Input: part model. Units: mm. Frame: model coordinates. A direction names the side the tool comes from. Coordinates: 2 decimals unless noted, no trailing zeros. Order: outer loops, then holes, each group sorted by start corner. A loop starts at its lowest first (then second) coordinate and runs counter-clockwise, first axis right, second up. Notation, with made-up numbers: (22.25, -25) -> (68.25, -25) arc R37 ccw to (68.25, 14) -> close; hole circle Ø11 at (-17.5, -34). An arc over 180 degrees is marked (long way). One line per question, with ' | ' between items.
```python
from build123d import *

# Parameters (mm, degrees)
F0_W      = 22.5
F0_H      = 11.8
F1_DEPTH  = 22.7
F2_W      = 4.7
F2_H      = 2.5
F3_DEPTH  = 11.8
F5_DEPTH  = 2.5
F7_DEPTH  = 2.5
F9_DEPTH  = 4
F10_R     = 2.3
F10_R_2   = 0.85
F11_DEPTH = 3.2
F13_DEPTH = 2


with BuildPart() as f1:
    # F0 (on Top) → F1 (new body)
    with BuildSketch(Plane.XY):
        with Locations((-42.3355284333, 9.1565789297)):
            Rectangle(F0_W, F0_H)
    extrude(amount=F1_DEPTH)

    # F2 (on face) → F3 (join)
    with BuildSketch(Plane.XZ.offset(-3.2565789297)):
        with Locations((-55.9355284333, 17.15)):
            Rectangle(F2_W, F2_H)
        with Locations((-28.7355284333, 17.15)):
            Rectangle(F2_W, F2_H)
    extrude(amount=-F3_DEPTH)

    # F4 (on face) → F5 (cut)
    with BuildSketch(Plane.XY.offset(18.4)):
        with BuildLine():
            Line((-58.2855284333, 8.5065789297), (-56.745462641, 8.5065789297))
            ThreePointArc((-56.745462641, 8.5065789297), (-54.9855284333, 9.1565789297), (-56.745462641, 9.8065789297))
            Line((-56.745462641, 9.8065789297), (-58.2855284333, 9.8065789297))
            Line((-58.2855284333, 9.8065789297), (-58.2855284333, 9.1565789297))
            Line((-58.2855284333, 9.1565789297), (-58.2855284333, 8.5065789297))
        make_face()
    extrude(amount=-F5_DEPTH, mode=Mode.SUBTRACT)

    # F6 (on face) → F7 (cut)
    with BuildSketch(Plane.XY.offset(18.4)):
        with BuildLine():
            Line((-26.3855284333, 9.8065789297), (-27.9255942256, 9.8065789297))
            ThreePointArc((-27.9255942256, 9.8065789297), (-29.6855284333, 9.1565789297), (-27.9255942256, 8.5065789297))
            Line((-27.9255942256, 8.5065789297), (-26.3855284333, 8.5065789297))
            Line((-26.3855284333, 8.5065789297), (-26.3855284333, 9.1565789297))
            Line((-26.3855284333, 9.1565789297), (-26.3855284333, 9.8065789297))
        make_face()
    extrude(amount=-F7_DEPTH, mode=Mode.SUBTRACT)

    # F8 (on face) → F9 (join)
    with BuildSketch(Plane.XY.offset(22.7)):
        with BuildLine():
            Line((-41.3855284333, 11.6565789297), (-42.341372747, 11.6565789297))
            ThreePointArc((-42.341372747, 11.6565789297), (-44.5185109103, 14.1345303165), (-47.6855284366, 15.0565789297))
            ThreePointArc((-47.6855284366, 15.0565789297), (-51.8574584435, 13.3285089376), (-53.5855284333, 9.1565789297))
            ThreePointArc((-53.5855284333, 9.1565789297), (-51.8574584423, 4.9846489207), (-47.6855284333, 3.2565789297))
            ThreePointArc((-47.6855284333, 3.2565789297), (-44.5185109089, 4.1786275439), (-42.341372747, 6.6565789297))
            Line((-42.341372747, 6.6565789297), (-41.3855284333, 6.6565789297))
            ThreePointArc((-41.3855284333, 6.6565789297), (-38.8855284333, 9.1565789297), (-41.3855284333, 11.6565789297))
        make_face()
    extrude(amount=F9_DEPTH)

    # F10 (on face) → F11 (join)
    with BuildSketch(Plane.XY.offset(26.7)):
        with Locations((-47.6855284333, 9.1565789297)):
            Circle(F10_R)
        with Locations((-47.6855284333, 9.1565789297)):
            Circle(F10_R_2, mode=Mode.SUBTRACT)
    extrude(amount=F11_DEPTH)

    # F12 (on face) → F13 (cut)
    with BuildSketch(Plane.YZ.offset(-31.0855284333)):
        Polygon((7.3565789297, 4.5), (9.1565789297, 4.5), (10.9565789297, 4.5), (10.9565789297, 5.7), (7.3565789297, 5.7), align=None)
    extrude(amount=-F13_DEPTH, mode=Mode.SUBTRACT)


solid = f1.part
```
1. Pin query (flat end, axial travel): pin 1 Ø2 at (x, y) = (-32.5, 9) entering from +Z; pin 2 Ø0.5 at (x, y) = (-47.5, 9) entering from +Z; pin 3 Ø3 at (y, z) = (9, 6) entering from +X; pin 4 Ø1.5 at (x, z) = (-55, 8) entering from +Y. Return the tip coordinate at first contact, or that it passes through.
Recorded:
pin 1: stops at z = 22.7 | pin 2: stops at z = 26.7 | pin 3: stops at x = -31.09 | pin 4: passes through
2. Cut plane C-C, the plane y = 4.5. Return loops of the section in (x, z).
Recorded:
outline: (-58.29, 15.9) -> (-53.59, 15.9) -> (-53.59, 0) -> (-31.09, 0) -> (-31.09, 15.9) -> (-26.39, 15.9) -> (-26.39, 18.4) -> (-31.09, 18.4) -> (-31.09, 22.7) -> (-44.06, 22.7) -> (-44.06, 26.7) -> (-51.31, 26.7) -> (-51.31, 22.7) -> (-53.59, 22.7) -> (-53.59, 18.4) -> (-58.29, 18.4) -> close
3. Cut plane A-A, the plane z = 18. Return loops of the section in (x, y), and give its area (3 significant figures).
Recorded:
outline: (-58.29, 3.26) -> (-26.39, 3.26) -> (-26.39, 8.51) -> (-27.93, 8.51) arc R1 cw (long way) to (-27.93, 9.81) -> (-26.39, 9.81) -> (-26.39, 15.06) -> (-58.29, 15.06) -> (-58.29, 9.81) -> (-56.75, 9.81) arc R1 cw (long way) to (-56.75, 8.51) -> (-58.29, 8.51) -> close | area: 367 mm^2
4. Ray query, line 1 (X direction, y = 9.25, z = 27); line 2 (Z direction, x = -32.5, y = 9); line 3 (Z direction, x = -50, y = 7.25). Return the intervals inside material, ascending. Write a range as [from, to].
Recorded:
line 1: x = [-49.98, -48.53], [-46.84, -45.39] | line 2: z = [0, 4.5], [5.7, 22.7] | line 3: z = [0, 26.7]
5. Mould query, pull axis Y, two halves, no side actions, for faces 1 (the face through (-32, 7.357, 5)), 2 (the face through (-30, 9, 15.9)), 3 (the face through (-43, 15.057, 11)). Classes: released by +Y, released by -Y, zero draft, split by the parting line, or undercut.
Recorded:
face 1: undercut | face 2: zero draft | face 3: released by +Y
6. Cut plane B-B, the plane x = -56. Return loops of the section in (y, z).
Recorded:
outline: (3.26, 15.9) -> (8.16, 15.9) -> (8.16, 18.4) -> (3.26, 18.4) -> close; (10.16, 15.9) -> (15.06, 15.9) -> (15.06, 18.4) -> (10.16, 18.4) -> close
7. Cut plane D-D, the plane x = -34. Return loops of the section in (y, z), and give its area (3 significant figures).
Recorded:
outline: (3.26, 0) -> (15.06, 0) -> (15.06, 22.7) -> (3.26, 22.7) -> close | area: 268 mm^2
8. Access query for faces 4 (the face through (-58, 9.807, 17)), 5 (the face through (-56, 10.4, 18.4)), 6 (the face through (-32, 9, 4.5)). Directions: +Z, -Z, +X, -X, +Y, -Y. A direction counts if a zero-diameter tool reaches every point of the face in a straight line with its end or side. Return the directions, or none.
Recorded:
face 4: +Z, -Z, -X | face 5: +Z, -X, +Y, -Y | face 6: +X
